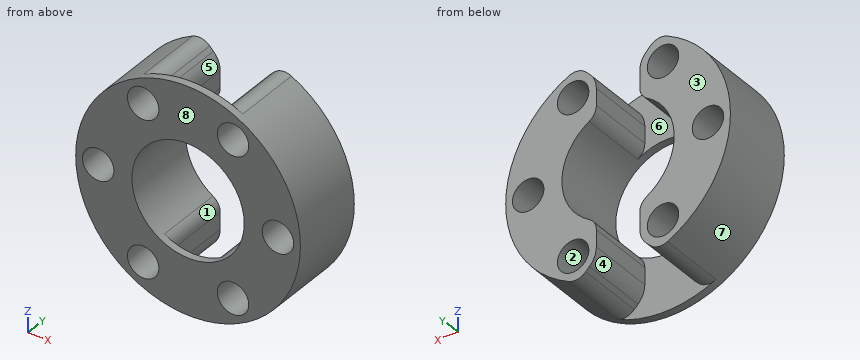
Autodesk Inventor part; units mm, degrees
ref_plane "YZ Plane" through (0, 0, 0) normal (1, 0, 0) x (0, 1, 0)
ref_plane "XZ Plane" through (0, 0, 0) normal (0, 1, 0) x (-1, 0, 0)
ref_plane "XY Plane" through (0, 0, 0) normal (0, 0, 1) x (1, 0, 0)
sketch "スケッチ1" plane through (0, 0, 0) normal (0, 1, 0) x (-1, 0, 0)
  circle A0 centre (0, 0) radius 15
  dimension "d0" = 30
extrude "押し出し1" add sketch "スケッチ1" along normal blind 10
sketch "スケッチ2" plane through (0, 10, 0) normal (0, 1, 0) x (1, 0, 0)
  circle A0 centre (0, 0) radius 12
  point P0 (-12, 0)
  point P1 (-6, -10.3923)
  point P2 (6, -10.3923)
  point P3 (12, 0)
  point P4 (6, 10.3923)
  point P5 (-6, 10.3923)
  dimension "d3" = 24
  dimension "d6" = 360
hole "穴1" at (-12, 10, 0) at (-6, 10, 10.3923) at (6, 10, 10.3923) at (12, 10, 0) at (6, 10, -10.3923) at (-6, 10, -10.3923) direction (0, -1, 0) diameter 4.2 end through all
sketch "スケッチ3" plane through (0, 10, 0) normal (0, 1, 0) x (1, 0, 0)
  circle A0 centre (0, 0) radius 7.5
  dimension "d15" = 15
extrude "押し出し2" cut sketch "スケッチ3" against normal blind 10
sketch "スケッチ4" plane through (0, 10, 0) normal (0, 1, 0) x (1, 0, 0)
  circle A0 centre (-6, -10.3923) radius 2.1
  circle A1 centre (6, -10.3923) radius 2.1
  line L0 (-6, -10.3923) -> (6, -10.3923)
  circle A2 centre (-6, -10.3923) radius 3.1
  circle A3 centre (6, -10.3923) radius 3.1
  line L1 (-2.9, -10.3923) -> (-2.9, -6.9166)
  circle A4 centre (0, 0) radius 7.5
  line L2 (2.9, -10.3923) -> (2.9, -6.9166)
  line L3 (-3.808, -12.5843) -> (-5.2681, -14.0445)
  circle A5 centre (0, 0) radius 15
  line L4 (3.808, -12.5843) -> (5.2681, -14.0445)
  line L5 (-15, 0) -> (0, 0)
  circle A6 centre (-6, 10.3923) radius 3.1
  circle A7 centre (6, 10.3923) radius 3.1
  line L6 (-2.9, 10.3923) -> (-2.9, 6.9166)
  line L7 (2.9, 10.3923) -> (2.9, 6.9166)
  line L8 (-3.808, 12.5843) -> (-5.2681, 14.0445)
  line L9 (3.808, 12.5843) -> (5.2681, 14.0445)
  circle A8 centre (0, 0) radius 7.5
  circle A9 centre (0, 0) radius 15
  point P0 (-5.2681, 14.0445)
  dimension "d18" = 1
  dimension "d19" = 1
  dimension "d20" = 135
extrude "押し出し3" cut sketch "スケッチ4" against normal blind 9 contours L1 A4 L2 L0 | L0 A3 L4 A5 L3 A2 | L6 A6 L8 A5 L9 A7 L7 A4
fillet "フィレット1" radius 2 8 edges at (5.2681, 5.5, -14.0445) (-5.2681, 5.5, -14.0445) (5.2681, 5.5, 14.0445) (-5.2681, 5.5, 14.0445) (-2.9, 5.5, -6.9166) (-2.9, 5.5, 6.9166) (2.9, 5.5, 6.9166) (2.9, 5.5, -6.9166)
sketch "スケッチ5" plane through (0, 1, 0) normal (0, 1, 0) x (1, 0, 0)
  arc A0 (-6.6047, -13.4677) -> (6.6047, -13.4677) centre (0, 0) ccw
  line L0 (-2.9, -10.3923) -> (-2.9, -8.1388)
  arc A1 (6.6047, -13.4677) -> (-6.6047, -13.4677) centre (0, 0) ccw
  circle A2 centre (0, 0) radius 15
  line L1 (-6.1706, -13.672) -> (6.1706, -13.672)
  arc A3 (4.3098, -13.0862) -> (6.6047, -13.4677) centre (5.724, -11.672) ccw
  line L2 (6.1706, -13.672) -> (-6.1706, -13.672)
  line L3 (-6.1706, -13.672) -> (-6.1706, -24.6433)
  line L4 (-6.1706, -24.6433) -> (6.1706, -24.6433)
  line L5 (6.1706, -24.6433) -> (6.1706, -13.672)
  line L6 (-6.1706, -24.6433) -> (-15.2853, -20.5296)
  line L7 (-15.2853, -20.5296) -> (-10.7439, -10.4675)
  line L8 (-6.1706, -13.672) -> (-11.1715, -11.4149)
  point P0 (-10.7439, -10.4675)
  dimension "d28" = 10
  dimension "d29" = 10
extrude "押し出し4" [suppressed]
sketch "スケッチ6" plane through (0, 1, 0) normal (0, 1, 0) x (1, 0, 0)
  line L0 (-15.6324, -20.1472) -> (-7.4753, -3.7413)
  line L1 (-14.742, -18.3563) -> (-2.1859, -24.5993)
  line L2 (6.6781, -24.5993) -> (-6.6781, -24.5993)
  line L3 (-6.6781, -24.5993) -> (-15.6324, -20.1472)
  line L4 (-10.7006, -22.5993) -> (6.6781, -22.5993)
  line L5 (6.6781, 0) -> (6.6781, -24.5993)
  line L6 (-15.6324, -20.1472) -> (-6.6781, -24.5993)
  line L7 (-6.6781, -24.5993) -> (6.6781, -24.5993)
  line L8 (0, -24.5993) -> (0, -22.5993)
  point P0 (0, 0)
  point P1 (-15, 0)
  point P2 (-15, 0)
  point P3 (-6.2084, -22.5993)
  dimension "d33" = 2
  dimension "d34" = 2
extrude "押し出し5" [suppressed]
properties part number "servoplate_forR2" material "アルミニウム 6061"
Check sheet for the modelled part. Datum: model origin and axes. Units: mm. Face numbers are marked on the shaded views. A direction names the side the tool comes from. Give positions to 0.01 mm unless a question says otherwise; leave off trailing zeros. Write each loop counter-clockwise with the first axis right and the second up, starting at its lowest first coordinate (ties: lowest second). Pieces come first, ordered by that corner, then holes. Notation, with made-up numbers: (-27, -39) - (-5, -39) arc R33 ccw to (-5, -2) - close; hole circle Ø2 at (68, -23.5). An arc over 180 degrees is marked (long way). Answer as a JSON object with one key per item and string values. Group by question number.
1) Sectioned sample at C-C (z = 2.75). Record the cut outline in (x, y), then the cut area to 3 significant figures.
2) Sectioned sample at A-A (x = 0). Record the cut outline in (y, z), then the cut area to 3 significant figures.
3) Sectioned sample at B-B (y = 0.5). Record the cut outline in (x, z).
4) Release check for a two-part mould opening along X. For the marked faces 6, 7 and 8 record: pulls with the +X half, pulls with the -X half, needs draft (parallel to the pull), parting line crosses it, or undercut.
5) Thickness scan on probe 1 along X at (y, z) = (6.5, 0); probe 2 along Z at (x, y) = (-6, 6); probe 3 along Z at (x, y) = (-5.25, 9). Record the ranges inside material, lowest first. Write a range as from..to.
6) Access from +Z, -Z, +X, -X, +Y, -Y to the whole of each face (thin tool, end or side, straight path). Record for the marked faces 1, 2, 3, 4 and 5.
7) Sectioned sample at D-D (y = 8). Give the number of separate pieces and of enclosed holes in the cut face, then the cut area to 3 significant figures.
8) Depth check by flat-ended pin: P1, Ø2.5, axis at y = 6, z = 9.5, coming from the -X side; P2, Ø3.5, axis at x = -6, z = 10.39, coming from the +Y side; P3, Ø2.5, axis at y = 6.5, z = -9, coming from the +X side; P4, Ø5, axis at x = -10, y = 6, coming from the -Z side. Enter the tip coordinate at first touch or a pass-through.
Geometry results:
{
 "1": {"outline": "(-14.75, 0) - (-6.98, 0) - (-6.98, 10) - (-14.75, 10) - close; (6.98, 0) - (14.75, 0) - (14.75, 10) - (6.98, 10) - close", "area": "155 mm^2"},
 "2": {"outline": "(0, -15) - (1, -15) - (1, -7.5) - (0, -7.5) - close; (0, 7.5) - (1, 7.5) - (1, 15) - (0, 15) - close", "area": "15.0 mm^2"},
 "3": {"outline": "circle Ø30 at (0, 0); hole circle Ø4.2 at (-12, 0); hole circle Ø4.2 at (-6, -10.39); hole circle Ø4.2 at (-6, 10.39); hole circle Ø15 at (0, 0); hole circle Ø4.2 at (6, -10.39); hole circle Ø4.2 at (6, 10.39); hole circle Ø4.2 at (12, 0)"},
 "4": {"face 6": "undercut", "face 7": "parting line crosses it", "face 8": "needs draft"},
 "5": {"probe 1": "x = -15..-14.1, -9.9..-7.5, 7.5..9.9, 14.1..15", "probe 2": "z = -13.65..-12.49, -8.29..-4.5, 4.5..8.29, 12.49..13.65", "probe 3": "z = -13.61..-12.35, -8.43..-5.36, 5.36..8.43, 12.35..13.61"},
 "6": {"face 1": "+Y", "face 2": "+Y, -Y", "face 3": "+Z, -Z, +X, -X, +Y", "face 4": "-Z, +Y", "face 5": "+Z, +Y"},
 "7": {"separate pieces": "2", "enclosed holes": "6", "area": "341 mm^2"},
 "8": {"P1": "stops at x = -12.53", "P2": "passes through", "P3": "stops at x = 12.84", "P4": "stops at z = -12.99"}
}
